from build123d import *

# Parameters (mm, degrees)
CUT_EXTRUDE1_DEPTH = 400
SKETCH3_R          = 33
SKETCH3_R_2        = 3.1000000000000028
CUT_EXTRUDE2_DEPTH = 40
SKETCH3_2_R        = 3.1000000000000028
CUT_EXTRUDE4_DEPTH = 588.2704126987336
SKETCH4_R          = 7.750000000000002
SKETCH4_R_2        = 7.749999999999998
SKETCH4_R_3        = 7.75
CUT_EXTRUDE5_DEPTH = 30
CUT_EXTRUDE6_START = -166.72
CUT_EXTRUDE6_DEPTH = 166.72
CUT_EXTRUDE7_START = -166.72
CUT_EXTRUDE7_DEPTH = 40
FILLET1_R          = 3
FILLET2_R          = 1


# Read off the part's stored shape, not the designer's step: Cut-Extrude7
with BuildPart() as part:
    # Sketch1 → Revolve1 (revolve)
    with BuildSketch(Plane.XY, mode=Mode.PRIVATE) as revolve1_sk:
        with BuildLine():
            Line((650.0000000000001, 78.36), (600.0000000000001, 78.35999999999999))
            add(Edge.make_bspline(
                [(200.00000000000358, 42.32828037010144), (208.17052038042252, 43.51395402277683), (225.68488706430128, 45.99527814756255), (252.5646252490451, 49.61720291886234), (288.8377795121088, 54.154525537406215), (326.32073414086074, 58.489281573967666), (363.84117713275197, 62.4863121261995), (401.3959942076804, 66.1465092198773), (438.98297125108434, 69.46060873551288), (476.60065297069735, 72.40710938265987), (509.54226569024473, 74.62869781075653), (537.7964811389767, 76.23350465282824), (560.2922621801154, 77.27545940077594), (575.1953567037801, 77.83264328043563), (587.2142250450652, 78.17300672656529), (594.5199761893905, 78.31035588184413), (598.173256760109, 78.35432466011183), (600.0000000000001, 78.35999999999999)],
                knots=[0.33782774337518406, 0.33782774337518406, 0.33782774337518406, 0.33782774337518406, 0.33782774337518406, 0.3922467059008778, 0.45442341660838875, 0.5166001272068571, 0.5787768404127641, 0.6409535517353824, 0.7031302632972144, 0.7653069754242735, 0.8274836869805778, 0.8896603985814769, 0.9207487548355946, 0.9518371110897123, 0.9759185555448562, 0.9879592777724281, 1, 1, 1, 1, 1], degree=4))
            Line((200.0000000000036, 42.32828037010143), (200, -7.43e-14))
            Line((200, 0), (776.72, 0))
            Line((776.72, 0), (776.72, 54))
            Line((776.72, 54), (650.0000000000001, 54))
            Line((650.0000000000001, 54), (650.0000000000001, 78.36))
        make_face()
    revolve(revolve1_sk.sketch.rotate(Axis((776.72, 0, 0), (-1, 0, 0)), 90), axis=Axis((776.72, 0, 0), (-1, 0, 0)))

    # Sketch2 → Cut-Extrude1 (cut)
    with BuildSketch(Plane(origin=(776.72, 0, 0), x_dir=(0, 0, -1), z_dir=(1, 0, 0))):
        with BuildLine():
            ThreePointArc((47.36738574096539, -16.010333165383813), (-35.35533905932756, 35.35533905932719), (16.01033316538431, -47.367385740965226))
            ThreePointArc((16.010333165384957, -47.36738574096489), (14.843408327061695, -43.77194076139418), (14.25549204864172, -40.03786890496388))
            ThreePointArc((14.25549204864269, -40.03786890496403), (30.05203820042843, -30.05203820042811), (40.037868904964185, -14.255492048642266))
            ThreePointArc((40.03786890496402, -14.255492048641287), (43.77194076139434, -14.843408327061226), (47.36738574096508, -16.01033316538445))
        make_face()
    extrude(amount=-CUT_EXTRUDE1_DEPTH, mode=Mode.SUBTRACT)

    # Sketch3 → Cut-Extrude2 (cut)
    with BuildSketch(Plane.ZY.offset(-200.00000000000273)):
        Circle(SKETCH3_R)
        with Locations((0, 20)):
            Circle(SKETCH3_R_2, mode=Mode.SUBTRACT)
        with Locations((0, -20)):
            Circle(SKETCH3_R_2, mode=Mode.SUBTRACT)
    extrude(amount=-CUT_EXTRUDE2_DEPTH, mode=Mode.SUBTRACT)

    # Sketch3<2> → Cut-Extrude4 (cut, through all)
    with BuildSketch(Plane.ZY.offset(-200.00000000000273)):
        with Locations((0, 20)):
            Circle(SKETCH3_2_R)
        with Locations((0, -20)):
            Circle(SKETCH3_2_R)
    extrude(amount=-CUT_EXTRUDE4_DEPTH, mode=Mode.SUBTRACT)

    # Sketch4 → Cut-Extrude5 (cut)
    with BuildSketch(Plane(origin=(650.0000000000001, 0, 0), x_dir=(0, 0, -1), z_dir=(1, 0, 0))):
        with Locations((0, 62.5)):
            Circle(SKETCH4_R)
        with Locations((62.499999999999986, -2.1825e-13)):
            Circle(SKETCH4_R_2)
        with Locations((-4.3715e-13, -62.5)):
            Circle(SKETCH4_R_3)
        with Locations((-62.49999999999999, 6.5573e-13)):
            Circle(SKETCH4_R_2)
    extrude(amount=-CUT_EXTRUDE5_DEPTH, mode=Mode.SUBTRACT)

    # Sketch2<3> → Cut-Extrude6 (cut)
    with BuildSketch(Plane(origin=(776.72, 0, 0), x_dir=(0, 0, -1), z_dir=(1, 0, 0)).offset(CUT_EXTRUDE6_START)):
        with BuildLine():
            ThreePointArc((18.674162122276517, -42.585510083018875), (19.845504593214095, -46.16550545726443), (21.667324002424465, -49.462380356933224))
            ThreePointArc((21.66732400242451, -49.46238035693348), (38.18376618407376, -38.18376618407337), (49.4623803569337, -21.667324002424003))
            ThreePointArc((49.46238035693346, -21.667324002423932), (46.16550545726464, -19.845504593213597), (42.58551008301907, -18.67416212227606))
            ThreePointArc((42.58551008301935, -18.674162122276265), (32.880465325174626, -32.88046532517429), (18.674162122276698, -42.58551008301916))
        make_face()
    extrude(amount=CUT_EXTRUDE6_DEPTH, mode=Mode.SUBTRACT)

    # Cut-Extrude7 outline → Cut-Extrude7 (cut)
    with BuildSketch(Plane(origin=(776.72, 0, 0), x_dir=(0, 0, -1), z_dir=(1, 0, 0)).offset(CUT_EXTRUDE7_START)):
        with BuildLine():
            ThreePointArc((49.462380357, -21.667324002), (38.183766184, -38.183766184), (21.667324002, -49.462380357))
            ThreePointArc((21.667324002, -49.462380357), (52.325901808, -52.325901808), (49.462380357, -21.667324002))
        make_face()
    extrude(amount=CUT_EXTRUDE7_DEPTH, mode=Mode.SUBTRACT)

    # Fillet1
    # the kernel refuses this fillet: 3 mm, written as the material it takes off along each edge
    with BuildSketch(Plane(origin=(783.0040750376627, -40.03786890496436, -14.255492048641756), x_dir=(0, 0.36048933664361255, -0.9327633344885766), z_dir=(-1, 0, 0))) as fillet1_piece_1:
        with BuildLine():
            CenterArc((2.3526530908588352, 2.998927692547355), FILLET1_R, 190.6958961912189, 77.77213613267259)
            ThreePointArc((-0.5952251863106816, 2.4421389866704493), (-0.3296065941102598, 1.2132715607510574), (0, 0))
            ThreePointArc((0, 0), (1.1362245041079626, 0.01519102224578455), (2.2724490082159248, 3e-17))
        make_face()
    extrude(amount=406.28407503766266, mode=Mode.SUBTRACT)
    with BuildSketch(Plane(origin=(783.0040750376628, -14.255492048641326, -40.03786890496452), x_dir=(0, -0.12935906708338796, -0.9915978175466682), z_dir=(-1, 0, 0))) as fillet1_piece_2:
        with BuildLine():
            CenterArc((2.356528139123201, 2.995883676075499), FILLET1_R, 195.22966173823434, 77.77213613267247)
            ThreePointArc((-0.5381137542877349, 2.207817492997983), (-0.25429790806270375, 1.1075059660548925), (0, 0))
            ThreePointArc((0, 0), (1.2568150075323716, -0.0329305913960081), (2.513630015064742, 0))
        make_face()
    extrude(amount=406.2840750376628, mode=Mode.SUBTRACT)
    with BuildSketch(Plane(origin=(650.0000000000001, -49.46238035693335, -21.667324002424486), x_dir=(0, -0.3710376913926641, 0.9286178070476584), z_dir=(1, 0, 0))) as fillet1_piece_3:
        with BuildLine():
            CenterArc((3.4382745469761065, -2.998391169718282), FILLET1_R, 88.12348720794618, 95.23374468145443)
            ThreePointArc((0.4434230907932443, -3.1740748496643687), (0.2853925875390597, -1.5781410862550613), (0, 0))
            ThreePointArc((0, 0), (1.7682554813020526, 0.0289589450709421), (3.5365109626041082, -1.1e-16))
        make_face()
    extrude(amount=135.56127740651016, mode=Mode.SUBTRACT)
    with BuildSketch(Plane(origin=(650.0000000000001, -21.667324002423964, -49.46238035693357), x_dir=(0, 0.9286178070476617, -0.3710376913926558), z_dir=(1, 0, 0))) as fillet1_piece_4:
        with BuildLine():
            CenterArc((3.438274546976126, 2.998391169718279), FILLET1_R, 176.64276811059946, 95.23374468145443)
            ThreePointArc((0.44342309079326614, 3.174074849664362), (0.28539258753907326, 1.5781410862550511), (0, 0))
            ThreePointArc((0, 0), (1.7682554813020637, -0.02895894507093817), (3.53651096260413, 5e-17))
        make_face()
    extrude(amount=135.56127740651016, mode=Mode.SUBTRACT)

    # Fillet2
    fillet2_edges = [part.edges().sort_by_distance(p)[0] for p in [
        (576.72, -47.36738574096506, -16.010333165384637),
        (576.72, -16.01033316538413, -47.36738574096523),
        (693.36, -18.67416212227616, -42.58551008301921),
        (693.36, -42.58551008301902, -18.674162122276606),
    ]]
    fillet(fillet2_edges, radius=FILLET2_R)


solid = part.part
Can you work these out from the model? Positions are in its coordinate system, mm. A direction names the side the tool comes from. Round coordinates to 2 decimals unless told otherwise and drop trailing zeros. Answer in a Markdown table with one row per item.
(1) Which directions (+Z, -Z, +X, -X, +Y, -Y) give clear straight access to the entire face, cutting with the end or side of a thin tool? Please do faces 1 (the face through (579.52, -30.216, -29.888)), 2 (the face through (624.65, 47.681, 62.184)), 3 (the face through (219.7, -12.6, 30.5)).
From the geometry:
| item | result |
|---|---|
| face 1 | +X |
| face 2 | +X, -X |
| face 3 | -X |
(2) For P1, Ø7, axis at y = -20, z = 0, coming from the -X side; P2, Ø10, axis at x = 709.5, y = 15, coming from the -Z side; P3, Ø10, axis at x = 694, z = 3, coming from the +Y side; P4, Ø5.5, axis at y = 20, z = 0, coming from the -X side, each with a flat end and sliding along its axis, tell me the tip position at first contact or that it passes through.
From the geometry:
| item | result |
|---|---|
| P1 | stops at x = 240 |
| P2 | stops at z = -53.07 |
| P3 | stops at y = 54 |
| P4 | passes through |
(3) Please list where these lines run through material, in increasing order: L1, parallel to Y at x = 641, z = 0; L2, parallel to Y at x = 254, z = -0.5; L3, parallel to Y at x = 230.5, z = 15.5. Write a range as from..to.
From the geometry:
| item | result |
|---|---|
| L1 | y = -78.36..-70.25, -54.75..-50, 50..54.75, 70.25..78.36 |
| L2 | y = -49.73..-23.06, -16.94..16.94, 23.06..49.73 |
| L3 | y = -43.96..-29.13, 29.13..43.96 |
(4) Suppose I cut it at A-A, the plane x = 345. Count the separate pieces of the cut face and the enclosed holes in it, plus the area to 3 significant figures.
From the geometry:
| item | result |
|---|---|
| separate pieces | 1 |
| enclosed holes | 2 |
| area | 11,400 mm2 |
(5) If we mould it in two halves opening along Y, with no side actions, what happens to faces 4 (the face through (712.47, 36.71, 39.6)), 5 (the face through (200, 22, -25)), 6 (the face through (240, 0, 0))? For each: released by +Y, released by -Y, zero draft, split by the parting line, or undercut.
From the geometry:
| item | result |
|---|---|
| face 4 | split by the parting line |
| face 5 | zero draft |
| face 6 | undercut |
